Check sheet for the modelled part. Datum: model origin and axes. Units: mm. Face numbers are marked on the shaded views. A direction names the side the tool comes from. Give positions to 0.01 mm unless a question says otherwise; leave off trailing zeros. Loops run counter-clockwise (first coordinate to the right, second up) from the corner with the lowest first, then second, coordinate; pieces in that order, holes last. Notation, with made-up numbers: M -34.75,24 L -24.75,24 A35 ccw -24.75,60 Z; hole C 35.5,-2.75 d9. An arc over 180 degrees is marked long. Put each result on its own line as item: value. Start each with the question number.
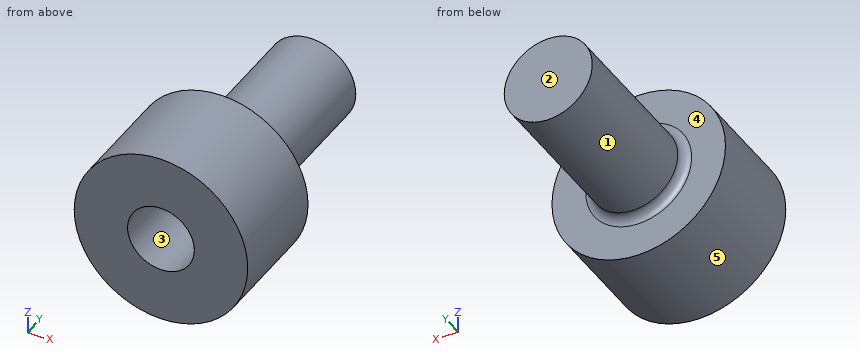
```python
from build123d import *

# Parameters (mm, degrees)
SKETCH1_R           = 4.875
SKETCH1_R_2         = 1.875
BOSS_EXTRUDE1_DEPTH = 6
SKETCH2_R           = 2.475
BOSS_EXTRUDE2_DEPTH = 9
FILLET1_R           = 0.5


with BuildPart() as part:
    # Sketch1 → Boss-Extrude1 (new body)
    with BuildSketch(Plane(origin=(0, 0, 0), x_dir=(1, 0, 0), z_dir=(0, 1, 0))):
        Circle(SKETCH1_R)
        Circle(SKETCH1_R_2, mode=Mode.SUBTRACT)
    extrude(amount=BOSS_EXTRUDE1_DEPTH)

    # Sketch2 → Boss-Extrude2 (add)
    with BuildSketch(Plane(origin=(0, 6, 0), x_dir=(1, 0, 0), z_dir=(0, 1, 0))):
        Circle(SKETCH2_R)
    extrude(amount=BOSS_EXTRUDE2_DEPTH)

    # Fillet1
    fillet1_edges = [part.edges().sort_by_distance(p)[0] for p in [
        (-2.475, 6, 0),
    ]]
    fillet(fillet1_edges, radius=FILLET1_R)


solid = part.part
```
Q1. Section check D-D, the plane y = 11. Record the cut outline in (x, z) (3 decimals).
Q2. Section check C-C, the plane y = 5.5. Record the cut outline in (x, z) (3 decimals).
Q3. Section check A-A, the plane x = 0. Record the cut outline in (y, z) (3 decimals).
Q4. Section check B-B, the plane z = 0. Record the cut outline in (x, y) (3 decimals), then the cut area to 3 significant figures.
Q5. Depth check by flat-ended pin: P1, Ø3, axis at y = 8.5, z = -3.5, coming from the +X side; P2, Ø4, axis at y = 10, z = 0.5, coming from the +X side (3 decimals); P3, Ø4, axis at y = 2, z = 3.5, coming from the -X side. Enter the tip coordinate at first touch or a pass-through.
Q6. Mould release check, pull along X, two halves, no side actions. Record for the marked faces 3, 4 and 5: pulls with the +X half, pulls with the -X half, needs draft (parallel to the pull), parting line crosses it, or undercut.
Q7. Thickness scan on line 1 along Z through (x, y) = (0, 3.95) (3 decimals); line 2 along Y through (x, z) = (2, -3). Record the ranges inside material, lowest first. Write a range as [from, to].
Q8. Access from +Z, -Z, +X, -X, +Y, -Y to the whole of each face (thin tool, end or side, straight path). Record for the marked faces 1 and 2.
Found:
1. outline: C 0,0 d4.95
2. outline: C 0,0 d9.75; hole C 0,0 d3.75
3. outline: M 0,-4.875 L 6,-4.875 L 6,-2.975 A0.5 cw 6.5,-2.475 L 15,-2.475 L 15,2.475 L 6.5,2.475 A0.5 cw 6,2.975 L 6,4.875 L 0,4.875 L 0,1.875 L 6,1.875 L 6,-1.875 L 0,-1.875 Z
4. outline: M -4.875,0 L -1.875,0 L -1.875,6 L 1.875,6 L 1.875,0 L 4.875,0 L 4.875,6 L 2.975,6 A0.5 cw 2.475,6.5 L 2.475,15 L -2.475,15 L -2.475,6.5 A0.5 cw -2.975,6 L -4.875,6 Z
4. area: 80.7 mm^2
5. P1: stops at x = 1.46
5. P2: stops at x = 2.475
5. P3: stops at x = -4.64
6. face 3: undercut
6. face 4: needs draft
6. face 5: parting line crosses it
7. line 1: z = [-4.875, -1.875], [1.875, 4.875]
7. line 2: y = [0, 6]
8. face 1: +Y
8. face 2: +Z, -Z, +X, -X, +Y
